from build123d import *

# Parameters (mm, degrees)
SKETCH_1_R      = 6
SKETCH_1_R_2    = 10
SKETCH_1_R_3    = 1.55
EXTRUDE_1_DEPTH = 7
FILLET_1_R      = 2


with BuildPart() as part:
    # 草图1 → 凸台-拉伸1 (new body)
    with BuildSketch(Plane.XY):
        with BuildLine():
            Line((25.733333333, -15.420621114), (-2.133333333, -7.710310557))
            ThreePointArc((-2.133333333, -7.710310557), (-8, 0), (-2.133333333, 7.710310557))
            Line((-2.133333333, 7.710310557), (25.733333333, 15.420621114))
            ThreePointArc((25.733333333, 15.420621114), (46, 0), (25.733333333, -15.420621114))
        make_face()
        Circle(SKETCH_1_R, mode=Mode.SUBTRACT)
        with Locations((30, 0)):
            Circle(SKETCH_1_R_2, mode=Mode.SUBTRACT)
        with Locations((30, -12.5)):
            Circle(SKETCH_1_R_3, mode=Mode.SUBTRACT)
        with Locations((21.161165235, -8.838834765)):
            Circle(SKETCH_1_R_3, mode=Mode.SUBTRACT)
        with Locations((17.5, 0)):
            Circle(SKETCH_1_R_3, mode=Mode.SUBTRACT)
        with Locations((21.161165235, 8.838834765)):
            Circle(SKETCH_1_R_3, mode=Mode.SUBTRACT)
        with Locations((30, 12.5)):
            Circle(SKETCH_1_R_3, mode=Mode.SUBTRACT)
        with Locations((38.838834765, 8.838834765)):
            Circle(SKETCH_1_R_3, mode=Mode.SUBTRACT)
        with Locations((42.5, 0)):
            Circle(SKETCH_1_R_3, mode=Mode.SUBTRACT)
        with Locations((38.838834765, -8.838834765)):
            Circle(SKETCH_1_R_3, mode=Mode.SUBTRACT)
        with BuildLine():
            Line((5.879001779, -6.814494705), (18.398019367, -10.27832892))
            ThreePointArc((18.398019367, -10.27832892), (14.5, 0), (18.398019367, 10.27832892))
            Line((18.398019367, 10.27832892), (5.879001779, 6.814494705))
            ThreePointArc((5.879001779, 6.814494705), (9, 0), (5.879001779, -6.814494705))
        make_face(mode=Mode.SUBTRACT)
    extrude(amount=EXTRUDE_1_DEPTH)

    # 圆角1
    fillet_1_edges = [part.edges().sort_by_distance(p)[0] for p in [
        (5.879001779, 6.814494705, 3.5),
        (5.879001779, -6.814494705, 3.5),
        (18.398019367, -10.27832892, 3.5),
        (18.398019367, 10.27832892, 3.5),
    ]]
    fillet(fillet_1_edges, radius=FILLET_1_R)


solid = part.part
Here's how the part is built. I have some questions about the finished solid (model axes, mm). A direction names the side the tool comes from. Coordinates: 2 decimals unless noted, no trailing zeros. Order: outer loops, then holes, each group sorted by start corner. A loop starts at its lowest first (then second) coordinate and runs counter-clockwise, first axis right, second up. Notation, with made-up numbers: M -8.5,-1.75 L 48.5,-1.75 A13 ccw 48.5,9.25 Z; hole C 33,36.5 d3. An arc over 180 degrees is marked long. Answer as CSV lines item,"result".
Item 1: We'd pull the mould along X, two halves only. Please class faces 3 (the face through (19.4, 0.2, 7)), 4 (the face through (16.27, -0.94, 3.45)), 5 (the face through (-8, 0, 3)), 6 (the face through (46, 0, 3)): +X half, -X half, draft (parallel to the pull), parting line (faces both ways), or undercut.
Results found:
face 3,"draft"
face 4,"undercut"
face 5,"-X half"
face 6,"parting line"
Item 2: For pin 1 (1.9 mm diameter, centred on x = 21.16, y = -8.84, fed in from -Z), with a flat end and sliding along its axis, tell me the tip position at first contact or that it passes through.
Results found:
pin 1,"through"
Item 3: On a 3-axis mill with a long thin cutter (end or side, diameter ignored), from which of +Z, -Z, +X, -X, +Y, -Y can I reach the whole of each face in a straight line? I mean faces 1 (the face through (19.4, 0.2, 0)), 2 (the face through (7.531, -6.426, 3.549)). Say none if no direction works.
Results found:
face 1,"-Z, +X, -X, +Y, -Y"
face 2,"+Z, -Z"
Item 4: If I drill on line 1 (X direction, y = -4, z = 2.5); line 2 (Y direction, x = 38, z = 2); line 3 (X direction, y = -2.5, z = 2.5), over which ranges is the centre line in solid material (lowest first)?
Results found:
line 1,"-6.93 to -4.47, 4.47 to 8.06, 15.03 to 20.83, 39.17 to 45.49"
line 2,"-13.86 to -10.14, -7.54 to -6, 6 to 7.54, 10.14 to 13.86"
line 3,"-7.6 to -5.45, 5.45 to 8.65, 14.7 to 20.32, 39.68 to 45.8"
Item 5: Imagine slicing it at C-C on x = 17.5. Write out the boundary of the cut face in (y, z).
Results found:
outline,"M -13.14,0 L -1.55,0 L -1.55,7 L -13.14,7 Z; M 1.55,0 L 13.14,0 L 13.14,7 L 1.55,7 Z"
Item 6: Imagine slicing it at B-B on x = 30. Write out the boundary of the cut face in (y, z).
Results found:
outline,"M -16,0 L -14.05,0 L -14.05,7 L -16,7 Z; M -10.95,0 L -10,0 L -10,7 L -10.95,7 Z; M 10,0 L 10.95,0 L 10.95,7 L 10,7 Z; M 14.05,0 L 16,0 L 16,7 L 14.05,7 Z"
Item 7: Imagine slicing it at A-A on y = 0. Write out the boundary of the cut face in (x, z).
Results found:
outline,"M -8,0 L -6,0 L -6,7 L -8,7 Z; M 6,0 L 9,0 L 9,7 L 6,7 Z; M 14.5,0 L 15.95,0 L 15.95,7 L 14.5,7 Z; M 19.05,0 L 20,0 L 20,7 L 19.05,7 Z; M 40,0 L 40.95,0 L 40.95,7 L 40,7 Z; M 44.05,0 L 46,0 L 46,7 L 44.05,7 Z"
Item 8: Imagine slicing it at D-D on y = 12.5. Write out the boundary of the cut face in (x, z), plus the area to 3 significant figures.
Results found:
outline,"M 15.18,0 L 28.45,0 L 28.45,7 L 15.18,7 Z; M 31.55,0 L 39.99,0 L 39.99,7 L 31.55,7 Z"
area,"152 mm2"
